Read the model definition and answer for the solid it produces. Units are mm, in the model's axes. Face numbers are marked on the shaded views. A direction names the side the tool comes from. Give positions to 0.01 mm unless a question says otherwise; leave off trailing zeros. Write each loop counter-clockwise with the first axis right and the second up, starting at its lowest first coordinate (ties: lowest second). Pieces come first, ordered by that corner, then holes. Notation, with made-up numbers: (46, -33.75) - (68, -33.75) arc R9 cw to (68, -26.75) - close; hole circle Ø11 at (23.25, 8.5). An arc over 180 degrees is marked (long way). Answer as CSV lines item,"result".
```python
from build123d import *

# Parameters (mm, degrees)
F1_DEPTH = 2336.8
F2_SIZE  = 190.5
F3_R     = 101.6


with BuildPart() as f1:
    # F0 (on Front) → F1 (new body)
    with BuildSketch(Plane.XZ):
        Polygon((0, 0), (-406.4, 0), (-406.4, -25.4), (-101.6, -25.4), (-101.6, -152.4), (0, -152.4), align=None)
    extrude(amount=-F1_DEPTH)

    # F2
    f2_edges = [f1.edges().sort_by_distance(p)[0] for p in [
        (-406.4, 2336.8, -12.7),
    ]]
    chamfer(f2_edges, length=F2_SIZE)

    # F3
    f3_edges = [f1.edges().sort_by_distance(p)[0] for p in [
        (-406.4, 2146.3, -12.7),
        (-406.4, 0, -12.7),
    ]]
    fillet(f3_edges, radius=F3_R)


solid = f1.part
```
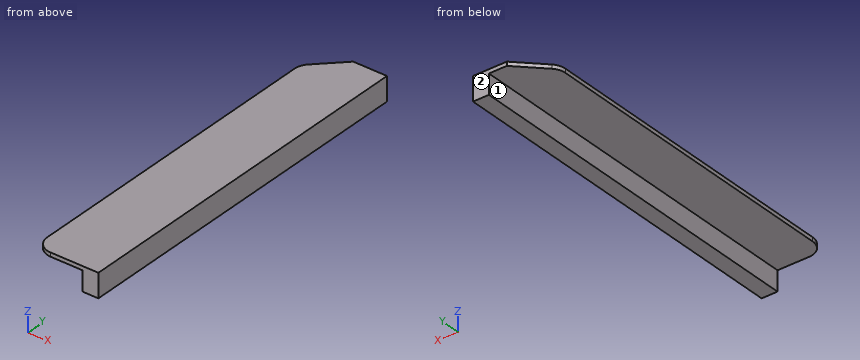
(1) For the marked faces 1 and 2, determine the directions among +Z, -Z, +X, -X, +Y, -Y from which every point of the face is accessible in a straight line to the end or side of a thin tool.
Worked out:
face 1,"-Z, -X, +Y, -Y"
face 2,"+Z, -Z, +X, -X, +Y"
(2) A cutting plane is placed at B-B (z = -81.5). Write down the section's boundary in (x, y).
Worked out:
outline,"(-101.6, 0) - (0, 0) - (0, 2336.8) - (-101.6, 2336.8) - close"
(3) A cutting plane is placed at A-A (y = 2056). Write down the section's boundary in (x, z), and give its area (3 significant figures).
Worked out:
outline,"(-406.4, -25.4) - (-101.6, -25.4) - (-101.6, -152.4) - (0, -152.4) - (0, 0) - (-406.4, 0) - close"
area,"23,200 mm^2"
(4) A cutting plane is placed at C-C (x = -126). Write down the section's boundary in (y, z), and give its area (3 significant figures).
Worked out:
outline,"(0, -25.4) - (2336.8, -25.4) - (2336.8, 0) - (0, 0) - close"
area,"59,400 mm^2"
(5) Find the intervals of material crossed by L1, parallel to X at y = 863, z = -66; L2, parallel to Z at x = -283.5, y = 1771; L3, parallel to Y at x = -256.5, z = -15, in increasing order.
Worked out:
L1,"x = -101.6 to 0"
L2,"z = -25.4 to 0"
L3,"y = 0 to 2296.2"
